Design review of the part built by this model. Coordinates are the model's own, in mm. Give positions to 0.01 mm unless a question says otherwise; leave off trailing zeros. Answer as a JSON object with one key per item and string values.
```python
from build123d import *

# Parameters (mm, degrees)
SKETCH1_W           = 5
SKETCH1_H           = 3.175
SKETCH1_W_2         = 3.175
SKETCH1_H_2         = 5.08
BOSS_EXTRUDE1_DEPTH = 3.175


with BuildPart() as part:
    # Sketch1 → Boss-Extrude1 (new body)
    with BuildSketch(Plane(origin=(0, 0, 0), x_dir=(1, 0, 0), z_dir=(0, 1, 0))):
        Polygon((-34.46085268, -83.030846574), (-34.46085268, -79.855846574), (-29.46085268, -79.855846574), (-29.46085268, -83.030846574), (-24.46085268, -83.030846574), (-24.46085268, -79.855846574), (-19.46085268, -79.855846574), (-19.46085268, -83.030846574), (-14.46085268, -83.030846574), (-14.46085268, -79.855846574), (-9.46085268, -79.855846574), (-9.46085268, -83.030846574), (-4.46085268, -83.030846574), (-4.46085268, -79.855846574), (0.53914732, -79.855846574), (0.53914732, -83.030846574), (5.53914732, -83.030846574), (5.53914732, -79.855846574), (10.53914732, -79.855846574), (10.53914732, -83.030846574), (15.53914732, -83.030846574), (15.53914732, -79.855846574), (20.53914732, -79.855846574), (20.53914732, -83.030846574), (25.53914732, -83.030846574), (25.53914732, -79.855846574), (30.53914732, -79.855846574), (30.53914732, -83.030846574), (74.87414732, -83.030846574), (74.87414732, 84.926653426), (30.53914732, 84.926653426), (30.53914732, 81.751653426), (25.53914732, 81.751653426), (25.53914732, 84.926653426), (20.53914732, 84.926653426), (20.53914732, 81.751653426), (15.53914732, 81.751653426), (15.53914732, 84.926653426), (10.53914732, 84.926653426), (10.53914732, 81.751653426), (5.53914732, 81.751653426), (5.53914732, 84.926653426), (0.53914732, 84.926653426), (0.53914732, 81.751653426), (-4.46085268, 81.751653426), (-4.46085268, 84.926653426), (-9.46085268, 84.926653426), (-9.46085268, 81.751653426), (-14.46085268, 81.751653426), (-14.46085268, 84.926653426), (-19.46085268, 84.926653426), (-19.46085268, 81.751653426), (-24.46085268, 81.751653426), (-24.46085268, 84.926653426), (-29.46085268, 84.926653426), (-29.46085268, 81.751653426), (-34.46085268, 81.751653426), (-34.46085268, 84.926653426), (-78.79585268, 84.926653426), (-78.79585268, -83.030846574), align=None)
        with Locations((-21.96085268, 54.764153426)):
            Rectangle(SKETCH1_W, SKETCH1_H, mode=Mode.SUBTRACT)
        with Locations((-31.96085268, 54.764153426)):
            Rectangle(SKETCH1_W, SKETCH1_H, mode=Mode.SUBTRACT)
        with Locations((-11.96085268, 54.764153426)):
            Rectangle(SKETCH1_W, SKETCH1_H, mode=Mode.SUBTRACT)
        with Locations((-1.96085268, 54.764153426)):
            Rectangle(SKETCH1_W, SKETCH1_H, mode=Mode.SUBTRACT)
        with Locations((8.03914732, 54.764153426)):
            Rectangle(SKETCH1_W, SKETCH1_H, mode=Mode.SUBTRACT)
        with Locations((18.03914732, 54.764153426)):
            Rectangle(SKETCH1_W, SKETCH1_H, mode=Mode.SUBTRACT)
        with Locations((28.03914732, 54.764153426)):
            Rectangle(SKETCH1_W, SKETCH1_H, mode=Mode.SUBTRACT)
        with Locations((-21.96085268, -52.868346574)):
            Rectangle(SKETCH1_W, SKETCH1_H, mode=Mode.SUBTRACT)
        with Locations((-31.96085268, -52.868346574)):
            Rectangle(SKETCH1_W, SKETCH1_H, mode=Mode.SUBTRACT)
        with Locations((-11.96085268, -52.868346574)):
            Rectangle(SKETCH1_W, SKETCH1_H, mode=Mode.SUBTRACT)
        with Locations((-1.96085268, -52.868346574)):
            Rectangle(SKETCH1_W, SKETCH1_H, mode=Mode.SUBTRACT)
        with Locations((8.03914732, -52.868346574)):
            Rectangle(SKETCH1_W, SKETCH1_H, mode=Mode.SUBTRACT)
        with Locations((18.03914732, -52.868346574)):
            Rectangle(SKETCH1_W, SKETCH1_H, mode=Mode.SUBTRACT)
        with Locations((28.03914732, -52.868346574)):
            Rectangle(SKETCH1_W, SKETCH1_H, mode=Mode.SUBTRACT)
        with Locations((-54.34835268, 21.267903426)):
            Rectangle(SKETCH1_W_2, SKETCH1_H_2, mode=Mode.SUBTRACT)
        with Locations((-54.34835268, 31.427903426)):
            Rectangle(SKETCH1_W_2, SKETCH1_H_2, mode=Mode.SUBTRACT)
        with Locations((-54.34835268, 11.107903426)):
            Rectangle(SKETCH1_W_2, SKETCH1_H_2, mode=Mode.SUBTRACT)
        with Locations((-54.34835268, 0.947903426)):
            Rectangle(SKETCH1_W_2, SKETCH1_H_2, mode=Mode.SUBTRACT)
        with Locations((-54.34835268, -9.212096574)):
            Rectangle(SKETCH1_W_2, SKETCH1_H_2, mode=Mode.SUBTRACT)
        with Locations((-54.34835268, -19.372096574)):
            Rectangle(SKETCH1_W_2, SKETCH1_H_2, mode=Mode.SUBTRACT)
        with Locations((-54.34835268, -29.532096574)):
            Rectangle(SKETCH1_W_2, SKETCH1_H_2, mode=Mode.SUBTRACT)
        with Locations((50.42664732, -29.532096574)):
            Rectangle(SKETCH1_W_2, SKETCH1_H_2, mode=Mode.SUBTRACT)
        with Locations((50.42664732, -19.372096574)):
            Rectangle(SKETCH1_W_2, SKETCH1_H_2, mode=Mode.SUBTRACT)
        with Locations((50.42664732, -9.212096574)):
            Rectangle(SKETCH1_W_2, SKETCH1_H_2, mode=Mode.SUBTRACT)
        with Locations((50.42664732, 0.947903426)):
            Rectangle(SKETCH1_W_2, SKETCH1_H_2, mode=Mode.SUBTRACT)
        with Locations((50.42664732, 11.107903426)):
            Rectangle(SKETCH1_W_2, SKETCH1_H_2, mode=Mode.SUBTRACT)
        with Locations((50.42664732, 21.267903426)):
            Rectangle(SKETCH1_W_2, SKETCH1_H_2, mode=Mode.SUBTRACT)
        with Locations((50.42664732, 31.427903426)):
            Rectangle(SKETCH1_W_2, SKETCH1_H_2, mode=Mode.SUBTRACT)
    extrude(amount=BOSS_EXTRUDE1_DEPTH)


solid = part.part
```
(1) Clearance check with a flat-ended pin moving along its axis: pin 1 (1 mm diameter, centred on x = 28, y = 2, fed in from -Z). State where the tip first meets the part, or that it passes through.
Here are the results:
{"pin 1": "stops at z = -81.75"}
(2) For line 1 along X through (y, z) = (0.2, 31); line 2 along Z through (x, y) = (6.5, 2.2), list the stretches that pass through material, from the lowest coordinate up.
Here are the results:
{"line 1": "x = -78.8 to -55.94, -52.76 to 48.84, 52.01 to 74.87", "line 2": "z = -81.75 to -56.35, -53.18 to 51.28, 54.46 to 79.86"}
(3) We need section A-A, the plane y = 0.8. Give the number of separate pieces and of enclosed holes in the cut face, then the cut area to 3 significant figures.
Here are the results:
{"separate pieces": "1", "enclosed holes": "28", "area": "25,100 mm²"}
